Geometry check sheet. Reference: the model listing, model coordinates, mm. A direction names the side the tool comes from. Round coordinates to 2 decimals unless told otherwise and drop trailing zeros. Order: outer loops, then holes, each group sorted by start corner. A loop starts at its lowest first (then second) coordinate and runs counter-clockwise, first axis right, second up.
(1) Set-up check for faces 5 (the face through (-3.01, 17.15, 44.93)), 6 (the face through (-2.85, -16.99, 44.93)), 7 (the face through (20, 0, 5)), 8 (the face through (0, 0, 5)), 9 (the face through (-10, 0, 40)): record each of +Z, -Z, +X, -X, +Y, -Y from which the full face is reachable in a straight line by a thin tool's end or side.
(2) Go/stop test with flat-tipped pins: pin 1 (4 mm diameter, centred on y = -6, z = 16, fed in from +X); pin 2 (8 mm diameter, centred on y = 2, z = 6.5, fed in from +X); pin 3 (6 mm diameter, centred on y = -4, z = 30.5, fed in from +X). Record where each tip stops, or that it passes through.
(3) Material ranges on line 1 along Z through (x, y) = (-3.5, -17); line 2 along Z through (x, y) = (10, -7.5); line 3 along Z through (x, y) = (-11, -12), recorded low to high.
(4) Sectioned sample at A-A (y = 0). Record the boundary of the cut face in (x, z), plus the area to 3 significant figures.
(5) Release check for a two-part mould opening along Z. For faces 1 (the face through (-20, 0, 30)), 2 (the face through (-15, 0, 50)), 3 (the face through (-22, -20, 25)), 4 (the face through (-5, 0, 0)) record: +Z half, -Z half, draft (parallel to the pull), parting line (faces both ways), or undercut.
(6) Sectioned sample at D-D (z = 34). Record the boundary of the cut face in (x, y), plus the area to 3 significant figures.
(7) Sectioned sample at C-C (y = 7). Record the boundary of the cut face in (x, z) (3 decimals).
(8) Sectioned sample at B-B (x = 7.5). Record the boundary of the cut face in (y, z).
Autodesk Fusion 360 part; units mm, degrees
sketch "Sketch1" plane through (0, 0, 0) normal (0, 1, 0) x (1, 0, 0)
  line L0 (0, 0) -> (-30, 0)
  line L1 (-30, 0) -> (-30, -50)
  line L2 (-30, -50) -> (0, -50)
  line L3 (0, -50) -> (0, -40)
  line L4 (0, -40) -> (-20, -40)
  line L5 (-20, -40) -> (-20, -10)
  line L6 (-20, -10) -> (0, -10)
  line L7 (0, -10) -> (0, 0)
  dimension "d1" = 10
  dimension "d2" = 10
  dimension "d3" = 50
  dimension "d4" = 30
  dimension "d5" = 10
  dimension "d6" = 20
extrude "Extrude1" add sketch "Sketch1" along normal mid plane 40
sketch "Sketch2" plane through (0, 0, 0) normal (0, 0, -1) x (1, 0, 0)
  line L0 (-30, 20) -> (-30, -20)
  line L1 (-30, -20) -> (0, -20)
  line L2 (0, -20) -> (0, 20)
  line L3 (0, 20) -> (-30, 20)
  circle A0 centre (0, 0) radius 20
  circle A1 centre (0, 0) radius 10
  dimension "d9" = 20
extrude "Extrude2" add sketch "Sketch2" against normal blind 10 contours L2 A0 A1 picked at (16.5649, -1.4231)
extrude "Extrude3" cut sketch "Sketch2" against normal blind 15 contours L2 A1 picked at (1.8021, 2.8042)
fillet "Fillet1" radius 10 2 edges at (-20, 0, 10) (-30, 0, 0)
fillet "Fillet2" radius 10 2 edges at (0, -20, 45) (0, 20, 45)
Answer below:
1. face 5: +Z, +X, +Y
1. face 6: +Z, +X, -Y
1. face 7: +Z, -Z, +X
1. face 8: +Z, -Z
1. face 9: +X, +Y, -Y
2. pin 1: stops at x = -18
2. pin 2: stops at x = 20
2. pin 3: stops at x = -20
3. line 1: z = 0 to 10, 40 to 50
3. line 2: z = 0 to 10
3. line 3: z = 0 to 10.05, 40 to 50
4. outline: (-30, 10) arc R10 ccw to (-20, 0) - (0, 0) - (0, 10) - (-10, 10) arc R10 cw to (-20, 20) - (-20, 40) - (0, 40) - (0, 50) - (-30, 50) - close; (10, 0) - (20, 0) - (20, 10) - (10, 10) - close
4. area: 1,000 mm2
5. face 1: undercut
5. face 2: +Z half
5. face 3: draft
5. face 4: -Z half
6. outline: (-30, -20) - (-20, -20) - (-20, 20) - (-30, 20) - close
6. area: 400 mm2
7. outline: (-30, 10) arc R10 ccw to (-20, 0) - (0, 0) - (0, 10) - (-10, 10) arc R10 cw to (-20, 20) - (-20, 40) - (0, 40) - (0, 50) - (-30, 50) - close; (7.141, 0) - (18.735, 0) - (18.735, 10) - (7.141, 10) - close
8. outline: (-18.54, 0) - (-6.61, 0) - (-6.61, 10) - (-18.54, 10) - close; (6.61, 0) - (18.54, 0) - (18.54, 10) - (6.61, 10) - close
